The drawing under review shows one solid part. Ordinate dimensions are in mm from its lowest x, y, z. Round coordinates to 2 decimals unless told otherwise and drop trailing zeros. Order: outer loops, then holes, each group sorted by start corner. A loop starts at its lowest first (then second) coordinate and runs counter-clockwise, first axis right, second up. Notation, with made-up numbers: (37.25, -0.75) -> (45.25, -0.75) arc R16 cw to (45.25, 13.25) -> close; hole circle Ø1 at (-32, 56). An arc over 180 degrees is marked (long way). Put each result on its own line as item: value. Start each with the question number.
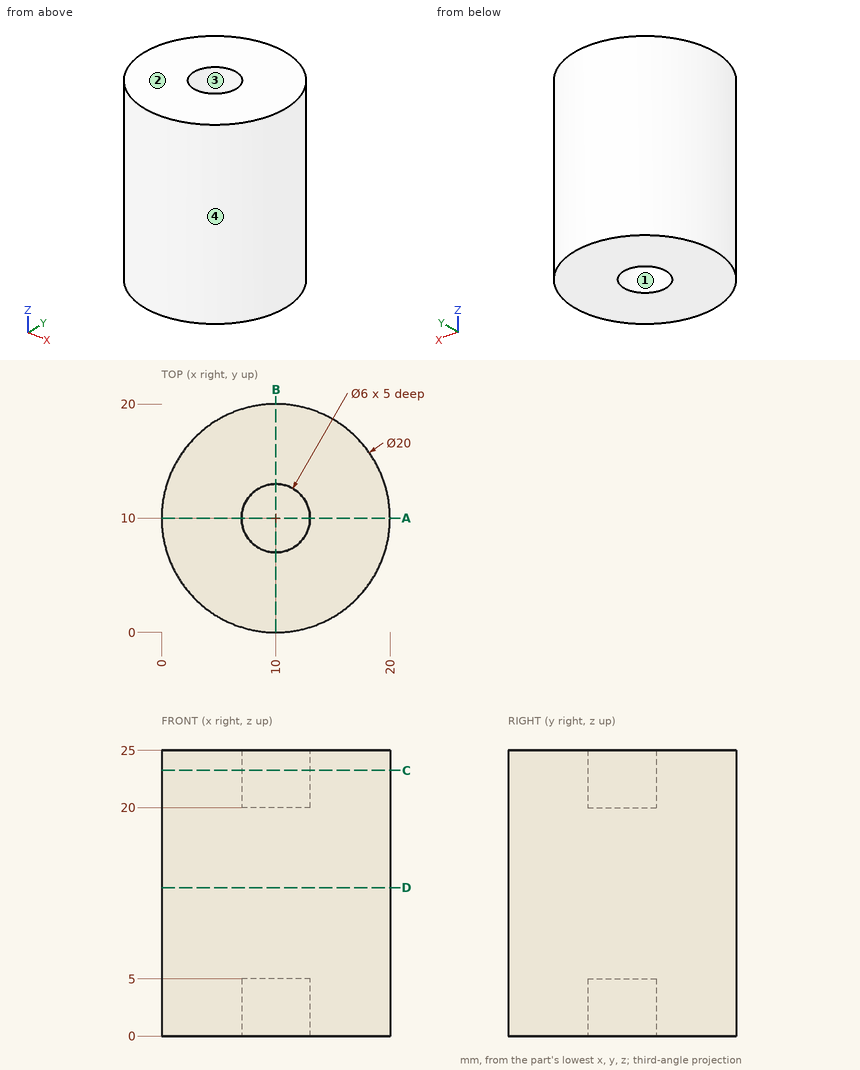
Item 1: Consider section A-A, the plane y = 10. Write out the cut boundary in (x, z).
Item 2: Consider section C-C, the plane z = 23.25. Write out the cut boundary in (x, y).
Item 3: Mouldability with a two-part tool opening along Y and no side actions: class the marked faces 1, 2, 3 and 4 as +Y half, -Y half, draft (parallel to the pull), parting line (faces both ways), or undercut.
Item 4: For L1, parallel to Y at x = 10, z = 1.4; L2, parallel to Z at x = 10.5, y = 10.5; L3, parallel to Y at x = 1.25, z = 16.5, list the stretches that pass through material, from the lowest coordinate up.
Item 5: Insertion check: pin 1 Ø1.8 at (x, y) = (9.5, 9) entering from +Z; pin 2 Ø2 at (x, z) = (8.5, 14.5) entering from -Y; pin 3 Ø4 at (y, z) = (15.5, 5) entering from -X. Each pin has a flat end and moves straight along its axis. Give the tip position at first contact, or say it passes through.
Item 6: Consider section D-D, the plane z = 13. Write out the cut boundary in (x, y).
Evaluation:
1. outline: (0, 0) -> (7, 0) -> (7, 5) -> (13, 5) -> (13, 0) -> (20, 0) -> (20, 25) -> (13, 25) -> (13, 20) -> (7, 20) -> (7, 25) -> (0, 25) -> close
2. outline: circle Ø20 at (10, 10); hole circle Ø6 at (10, 10)
3. face 1: undercut
3. face 2: draft
3. face 3: undercut
3. face 4: parting line
4. L1: y = 0 to 7, 13 to 20
4. L2: z = 5 to 20
4. L3: y = 5.16 to 14.84
5. pin 1: stops at z = 20
5. pin 2: stops at y = 0.01
5. pin 3: stops at x = 0.63
6. outline: circle Ø20 at (10, 10)
